Autodesk Fusion 360 part; units mm, degrees
sketch "Sketch1" plane through (0, 0, 0) normal (0, 0, 1) x (1, 0, 0)
  line L0 (-5.5, 6) -> (-9, -0.0622)
  line L1 (-9, -0.0622) -> (-5.5, -6.1244)
  line L2 (-5.5, -6.1244) -> (1.5, -6.1244)
  line L3 (1.5, -6.1244) -> (5, -0.0622)
  line L4 (5, -0.0622) -> (1.5, 6)
  line L5 (1.5, 6) -> (-5.5, 6)
  point P0 (-2, -0.0622)
extrude "Extrude1" add sketch "Sketch1" along normal blind 6
sketch "Sketch2" plane through (0, 0, 6) normal (0, 0, 1) x (-1, 0, 0)
  line L0 (-1.5, -6) -> (5.5, -6)
  line L1 (5.5, -6) -> (9, 0.0622)
  line L2 (9, 0.0622) -> (5.5, 6.1244)
  line L3 (5.5, 6.1244) -> (-1.5, 6.1244)
  line L4 (-1.5, 6.1244) -> (-5, 0.0622)
  line L5 (-5, 0.0622) -> (-1.5, -6)
  circle A0 centre (2, 0.0622) radius 5.25
  dimension "d3" = 10.5
extrude "Extrude2" add sketch "Sketch2" along normal blind 11.5 contours A0
fillet "Fillet1" radius 0.5 1 edges at (2.8947, -1.9607, 6)
sketch "Sketch3" plane through (0, 0, 17.5) normal (0, 0, 1) x (-1, 0, 0)
  circle A0 centre (2, 0.0622) radius 5.25
  circle A1 centre (2, 0.0622) radius 2
  dimension "d8" = 4
extrude "Extrude3" cut sketch "Sketch3" against normal blind 31.5 contours A1
chamfer "Chamfer1" distance 0.5 angle 45 2 edges at (-0.1353, -0.7854, 17.5) (2.8947, 1.8363, 17.5)
chamfer "Chamfer2" distance 0.5 angle 45 6 edges at (-2, -6.1244, 0) (-7.25, -3.0933, 0) (-7.25, 2.9689, 0) (-2, 6, 0) (3.25, 2.9689, 0) (3.25, -3.0933, 0)
CAD build for the part. Positions are in the model's coordinates, mm. A direction names the side the tool comes from. Coordinates: 2 decimals unless noted, no trailing zeros. Order: outer loops, then holes, each group sorted by start corner. A loop starts at its lowest first (then second) coordinate and runs counter-clockwise, first axis right, second up. Notation, with made-up numbers: (66, 86) -> (86, 86) arc R11 ccw to (86, 91) -> close; hole circle Ø5 at (-17, 74). An arc over 180 degrees is marked (long way). Use one line per item in the form item = value. Start each with the question number.
1) Band-saw the part on C-C on z = 10.75. Give the cut face in (x, y).
2) Drill centre lines: L1, parallel to Y at x = -2, z = 5; L2, parallel to Y at x = -2, z = 13.25; L3, parallel to X at y = 1.75, z = 2. Where is each one in solid material? Low to high. Write a range as [from, to].
3) Pull direction X, two halves, no side cores. Call faces 3 (the cylindrical face through (-1.74, -2.045, 8.619)), 4 (the cylindrical face through (-7.01, 1.51, 11.68)), 5 (the flat face through (-2, 6, 3)): +X half, -X half, draft (parallel to the pull), parting line (faces both ways), or undercut.
4) Band-saw the part on D-D on x = 4. Give the cut face in (y, z).
5) Drop flat-ended pins along their axis: pin 1 (2 mm diameter, centred on y = 2.5, z = 2.5, fed in from -X); pin 2 (8 mm diameter, centred on x = 0, z = 9, fed in from -Y); pin 3 (4 mm diameter, centred on y = -3.5, z = 6, fed in from +X); pin 4 (3 mm diameter, centred on y = 4.5, z = 11.5, fed in from +X). Give the stop position or say it passes through.
6) Band-saw the part on A-A on x = -2. Give the cut face in (y, z).
7) Tool access for faces 1 (the flat face through (4, 1, 6)), 2 (the flat face through (-4, 1, 0)): list every direction of +Z, -Z, +X, -X, +Y, -Y with a clear straight run to the whole face (end or side of a thin tool).
8) Band-saw the part on B-B on z = 4.5. Give the cut face in (x, y).
Entries:
q1.outline = circle Ø10.5 at (-2, -0.06); hole circle Ø4 at (-2, -0.06)
q2.L1 = [-6.12, -2.06], [1.94, 6]
q2.L2 = [-5.31, -2.06], [1.94, 5.19]
q2.L3 = [-7.95, -2.85], [-1.15, 3.95]
q3.face_3 = undercut
q3.face_4 = parting line
q3.face_5 = draft
q4.outline = (-1.79, 0.5) -> (-0.79, 0) -> (0.67, 0) -> (1.67, 0.5) -> (1.67, 6) -> (-1.79, 6) -> close
q5.pin_1 = -8.1
q5.pin_2 = -6.12
q5.pin_3 = 4.17
q5.pin_4 = 2.26
q6.outline = (-6.12, 0.5) -> (-5.62, 0) -> (-2.06, 0) -> (-2.06, 17) -> (-2.56, 17.5) -> (-4.81, 17.5) -> (-5.31, 17) -> (-5.31, 6.5) arc R0.5 cw to (-5.81, 6) -> (-6.12, 6) -> close; (1.94, 0) -> (5.5, 0) -> (6, 0.5) -> (6, 6) -> (5.69, 6) arc R0.5 cw to (5.19, 6.5) -> (5.19, 17) -> (4.69, 17.5) -> (2.44, 17.5) -> (1.94, 17) -> close
q7.face_1 = +Z
q7.face_2 = -Z, +X, -X, +Y, -Y
q8.outline = (-9, -0.06) -> (-5.5, -6.12) -> (1.5, -6.12) -> (5, -0.06) -> (1.5, 6) -> (-5.5, 6) -> close; hole circle Ø4 at (-2, -0.06)
